Geometry: see drawing. Coordinates: mm, zero at the bounding-box minimum. A direction names the side the tool comes from. Round coordinates to 2 decimals unless told otherwise and drop trailing zeros. Order: outer loops, then holes, each group sorted by start corner. A loop starts at its lowest first (then second) coordinate and runs counter-clockwise, first axis right, second up. Notation, with made-up numbers: (30, -33) -> (34, -33) arc R24 ccw to (34, -6) -> close; hole circle Ø6 at (-12.75, 78). An arc over 180 degrees is marked (long way). One line per item, written item: value. Start each with the question number.
1) Pin query (flat end, axial travel): P1, Ø1.5, axis at x = 16, z = 82, coming from the -Y side; P2, Ø2, axis at y = 1, z = 22, coming from the +X side; P3, Ø5, axis at x = 25, z = 48, coming from the +Y side. Return the tip coordinate at first contact, or that it passes through.
2) Section B-B (z = 73.5). Return the cut outline in (x, y).
3) Mould query, pull axis Z, two halves, no side actions, for the marked faces 3 and 4. Classes: pulls with the +Z half, pulls with the -Z half, needs draft (parallel to the pull), parting line crosses it, or undercut.
4) Ray query, L1, parallel to Z at x = 24, y = 2.15 (1 decimal); L2, parallel to Z at x = 47, y = 2.3 (1 decimal); L3, parallel to Z at x = 9.5, y = 3.3 (1 decimal). Return the intervals inside material, ascending.
5) Section A-A (y = 3.4). Return the cut outline in (x, z) (1 decimal), and give its area (3 significant figures).
6) Section C-C (x = 15.5). Return the cut outline in (y, z).
7) Reachability of the marked faces 1 and 2 from +Z, -Z, +X, -X, +Y, -Y: full face, straight path, thin tool, end or side. Return the list, or none.
8) Section D-D (z = 12). Return the cut outline in (x, y).
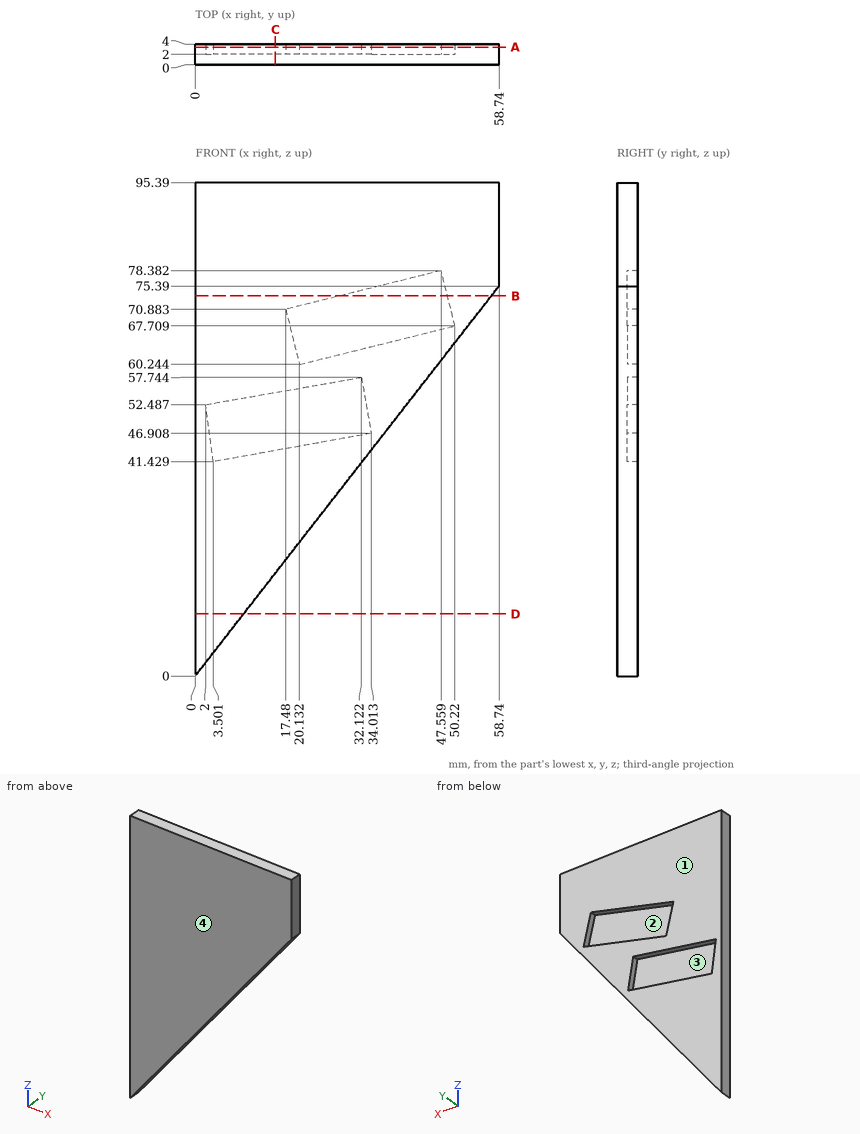
Findings:
1. P1: y = 0
1. P2: x = 17.92
1. P3: y = 2
2. outline: (0, 0) -> (57.27, 0) -> (57.27, 4) -> (48.78, 4) -> (48.78, 2) -> (27.98, 2) -> (27.98, 4) -> (0, 4) -> close
3. face 3: undercut
3. face 4: needs draft
4. L1: 30.8 to 45.1, 56.3 to 61.2, 72.5 to 95.4
4. L2: 60.3 to 66.9, 78.2 to 95.4
4. L3: 12.2 to 42.5, 53.8 to 95.4
5. outline: (0, 0) -> (58.7, 75.4) -> (58.7, 95.4) -> (0, 95.4) -> close; hole (2, 52.5) -> (3.5, 41.4) -> (34, 46.9) -> (32.1, 57.7) -> close; hole (17.5, 70.9) -> (20.1, 60.2) -> (50.2, 67.7) -> (47.6, 78.4) -> close
5. area: 2,710 mm2
6. outline: (0, 19.89) -> (4, 19.89) -> (4, 43.58) -> (2, 43.58) -> (2, 54.84) -> (4, 54.84) -> (4, 95.39) -> (0, 95.39) -> close
7. face 1: +Z, -Z, +X, -X, +Y
7. face 2: +Y
8. outline: (0, 0) -> (9.35, 0) -> (9.35, 4) -> (0, 4) -> close
